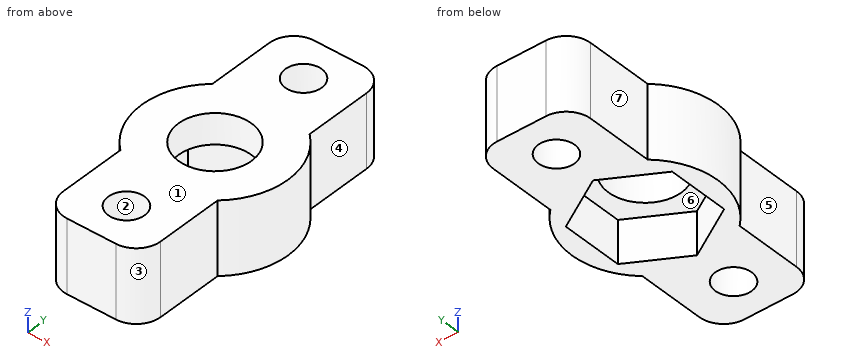
```python
from build123d import *

# Parameters (mm, degrees)
EXTRUDE_1_DEPTH           = 7.62
CUT_EXTRUDE_1_DEPTH       = 4.445
SKETCH_3_R                = 3.81
CUT_EXTRUDE_2_DEPTH       = 6.096
F_6_CLEARANCE_HOLE1_D     = 3.7973
F_6_CLEARANCE_HOLE1_DEPTH = 25.4
F_6_CLEARANCE_HOLE1_TIP   = 1.140824014


with BuildPart() as part:
    # 草图1 → 凸台-拉伸1 (new body)
    with BuildSketch(Plane.XY):
        with BuildLine():
            Line((-5.08, 12.7), (-5.08, 5.679612663))
            ThreePointArc((-5.08, 5.679612663), (-7.62, 0), (-5.08, -5.679612663))
            Line((-5.08, -5.679612663), (-5.08, -12.7))
            ThreePointArc((-5.08, -12.7), (-4.336051224, -14.496051224), (-2.54, -15.24))
            Line((-2.54, -15.24), (2.54, -15.24))
            ThreePointArc((2.54, -15.24), (4.336051224, -14.496051224), (5.08, -12.7))
            Line((5.08, -12.7), (5.08, -5.679612663))
            ThreePointArc((5.08, -5.679612663), (7.62, 0), (5.08, 5.679612663))
            Line((5.08, 5.679612663), (5.08, 12.7))
            ThreePointArc((5.08, 12.7), (4.336051224, 14.496051224), (2.54, 15.24))
            Line((2.54, 15.24), (-2.54, 15.24))
            ThreePointArc((-2.54, 15.24), (-4.336051224, 14.496051224), (-5.08, 12.7))
        make_face()
    extrude(amount=EXTRUDE_1_DEPTH)

    # 草图2 → 切除-拉伸1 (cut)
    with BuildSketch(Plane(origin=(0, 0, 0), x_dir=(-1, 0, 0), z_dir=(0, 0, -1))):
        Polygon((5.55625, 3.207902433), (0, 6.415804866), (-5.55625, 3.207902433), (-5.55625, -3.207902433), (0, -6.415804866), (5.55625, -3.207902433), align=None)
    extrude(amount=-CUT_EXTRUDE_1_DEPTH, mode=Mode.SUBTRACT)

    # 草图3 → 切除-拉伸2 (cut)
    with BuildSketch(Plane(origin=(0, 0, 4.445), x_dir=(-1, 0, 0), z_dir=(0, 0, -1))):
        Circle(SKETCH_3_R)
    extrude(amount=-CUT_EXTRUDE_2_DEPTH, mode=Mode.SUBTRACT)

    # #6 Clearance Hole1
    with Locations(Plane(origin=(0, 0, 0), x_dir=(-1, 0, 0), z_dir=(0, 0, -1))):
        with Locations((0, 10.922), (0, -10.922)):
            Hole(F_6_CLEARANCE_HOLE1_D / 2, depth=F_6_CLEARANCE_HOLE1_DEPTH)
            with Locations((0, 0, -(F_6_CLEARANCE_HOLE1_DEPTH + F_6_CLEARANCE_HOLE1_TIP / 2))):  # 118° drill point
                Cone(0, F_6_CLEARANCE_HOLE1_D / 2, F_6_CLEARANCE_HOLE1_TIP, mode=Mode.SUBTRACT)


solid = part.part
```
Could you check a few things on this model? Use its own coordinates, in mm. Face numbers are marked on the shaded views. A direction names the side the tool comes from. Give positions to 0.01 mm unless a question says otherwise; leave off trailing zeros. Loops run counter-clockwise (first coordinate to the right, second up) from the corner with the lowest first, then second, coordinate; pieces in that order, holes last. Notation, with made-up numbers: (52.25, 32) - (76.25, 32) arc R19 cw to (76.25, 56) - close; hole circle Ø3 at (25, 51). An arc over 180 degrees is marked (long way). Answer in a Markdown table with one row per item. Add a question column.
Q1. If we section it at B-B (x = -1.25): List the corners of the cut face in (y, z) for me (3 decimals), plus the area to 3 significant figures.
Q2. For pin 1 (2 mm diameter, centred on x = -3, y = -0.5, fed in from -Z) (3 decimals); pin 2 (1.5 mm diameter, centred on y = 1, z = 4, fed in from +X); pin 3 (2 mm diameter, centred on y = -10, z = 5, fed in from -X), each with a flat end and sliding along its axis, tell me the tip position at first contact or that it passes through.
Q3. If we section it at D-D (y = -8.5): List the corners of the cut face in (x, z) for me.
Q4. If we section it at C-C (z = 1.5): List the corners of the cut face in (x, y) for me.
Q5. If we section it at A-A (y = 0): List the corners of the cut face in (x, z) for me (3 decimals), plus the area to 3 significant figures.
Q6. Which directions (+Z, -Z, +X, -X, +Y, -Y) give clear straight access to the entire face, cutting with the end or side of a thin tool? Please do the marked faces 4, 5, 6 and 7.
Q7. Please list where these lines run through material, in increasing order: L1, parallel to Y at x = 0, z = 5.45; L2, parallel to X at y = -12, z = 5.75; L3, parallel to Y at x = 0.75, z = 3.5. Write a range as from..to.
Q8. We'd pull the mould along X, two halves only. Please class the marked faces 1, 2 and 3: +X half, -X half, draft (parallel to the pull), parting line (faces both ways), or undercut.
The answers:
| question | item | result |
|---|---|---|
| 1 | outline | (-15.24, 0) - (-12.351, 0) - (-12.351, 7.62) - (-15.24, 7.62) - close; (-9.493, 0) - (-5.694, 0) - (-5.694, 4.445) - (-3.599, 4.445) - (-3.599, 7.62) - (-9.493, 7.62) - close; (3.599, 4.445) - (5.694, 4.445) - (5.694, 0) - (9.493, 0) - (9.493, 7.62) - (3.599, 7.62) - close; (12.351, 0) - (15.24, 0) - (15.24, 7.62) - (12.351, 7.62) - close |
| 1 | area | 115 mm^2 |
| 2 | pin 1 | stops at z = 4.445 |
| 2 | pin 2 | stops at x = 7.62 |
| 2 | pin 3 | stops at x = -5.08 |
| 3 | outline | (-5.08, 0) - (5.08, 0) - (5.08, 7.62) - (-5.08, 7.62) - close |
| 4 | outline | (-5.08, -12.7) arc R2.54 ccw to (-2.54, -15.24) - (2.54, -15.24) arc R2.54 ccw to (5.08, -12.7) - (5.08, -5.68) arc R7.62 ccw to (5.08, 5.68) - (5.08, 12.7) arc R2.54 ccw to (2.54, 15.24) - (-2.54, 15.24) arc R2.54 ccw to (-5.08, 12.7) - (-5.08, 5.68) arc R7.62 ccw to (-5.08, -5.68) - close; hole (-5.56, -3.21) - (0, -6.42) - (5.56, -3.21) - (5.56, 3.21) - (0, 6.42) - (-5.56, 3.21) - close; hole circle Ø3.8 at (0, -10.92); hole circle Ø3.8 at (0, 10.92) |
| 5 | outline | (-7.62, 0) - (-5.556, 0) - (-5.556, 4.445) - (-3.81, 4.445) - (-3.81, 7.62) - (-7.62, 7.62) - close; (3.81, 4.445) - (5.556, 4.445) - (5.556, 0) - (7.62, 0) - (7.62, 7.62) - (3.81, 7.62) - close |
| 5 | area | 42.5 mm^2 |
| 6 | face 4 | +Z, -Z, +X, +Y |
| 6 | face 5 | +Z, -Z, -X, -Y |
| 6 | face 6 | -Z |
| 6 | face 7 | +Z, -Z, -X, +Y |
| 7 | L1 | y = -15.24..-12.82, -9.02..-3.81, 3.81..9.02, 12.82..15.24 |
| 7 | L2 | x = -5.08..-1.56, 1.56..5.08 |
| 7 | L3 | y = -15.24..-12.67, -9.18..-5.98, 5.98..9.18, 12.67..15.24 |
| 8 | face 1 | draft |
| 8 | face 2 | undercut |
| 8 | face 3 | +X half |
